Design review of the part shown in the three views and the two pictorial views. Dimensions are in mm from the part's minimum x, y and z. A direction names the side the tool comes from. Give positions to 0.01 mm unless a question says otherwise; leave off trailing zeros. Order: outer loops, then holes, each group sorted by start corner. A loop starts at its lowest first (then second) coordinate and runs counter-clockwise, first axis right, second up.
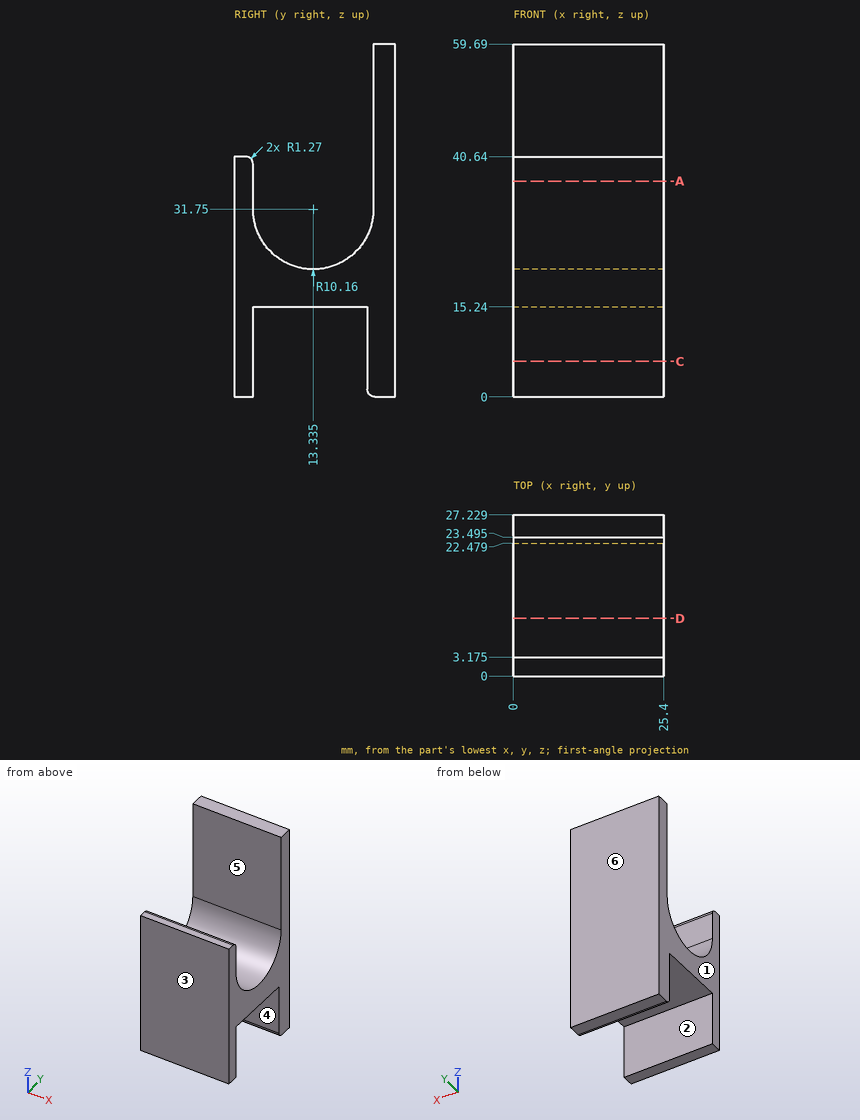
Item 1: Take a section at A-A (z = 36.5). Give the boundary of the cut face in (x, y) (1 decimal).
Values found:
outline: (0, 0) - (25.4, 0) - (25.4, 3.2) - (0, 3.2) - close; (0, 23.5) - (25.4, 23.5) - (25.4, 27.2) - (0, 27.2) - close
Item 2: Draft analysis for pull direction Y (two halves, no side actions). For the marked faces 1, 2 and 3, state which applies: released by +Y, released by -Y, zero draft, split by the parting line, or undercut.
Values found:
face 1: zero draft
face 2: undercut
face 3: released by -Y
Item 3: For the marked faces 4, 5 and 6, list the 3-axis set-ups (+Z, -Z, +X, -X, +Y, -Y) from which the entire face can be reached by the end or side of a thin tool; tool diameter is ignored.
Values found:
face 4: -Z, +X, -X
face 5: +Z, +X, -X
face 6: +Z, -Z, +X, -X, +Y
Item 4: For line 1 (Y direction, x = 22.25, z = 37.5) (1 decimal); line 2 (Y direction, x = 2.25, z = 13.5) (1 decimal); line 3 (Y direction, x = 10.75, z = 45.5) (1 decimal), list the stretches that pass through material, from the lowest coordinate up.
Values found:
line 1: y = 0 to 3.2, 23.5 to 27.2
line 2: y = 0 to 3.2, 22.5 to 27.2
line 3: y = 23.5 to 27.2
Item 5: Take a section at C-C (z = 6). Give the boundary of the cut face in (x, y) (1 decimal).
Values found:
outline: (0, 0) - (25.4, 0) - (25.4, 3.2) - (0, 3.2) - close; (0, 22.5) - (25.4, 22.5) - (25.4, 27.2) - (0, 27.2) - close
Item 6: Take a section at D-D (y = 9.75). Give the boundary of the cut face in (x, z), and give its area (3 significant figures).
Values found:
outline: (0, 15.24) - (25.4, 15.24) - (25.4, 22.24) - (0, 22.24) - close
area: 178 mm2
Item 7: Clearance check with flat-ended pins moving along their axes: pin 1 Ø5 at (x, y) = (6, 22) entering from +Z; pin 2 Ø0.6 at (x, y) = (17, 0.5) entering from +Z; pin 3 Ø1 at (x, y) = (12.5, 18) entering from +Z; pin 4 Ø6 at (x, y) = (8, 9.5) entering from -Z. State where each tip first meets the part, or that it passes through.
Values found:
pin 1: stops at z = 59.69
pin 2: stops at z = 40.64
pin 3: stops at z = 23
pin 4: stops at z = 15.24
